```python
from build123d import *

# Parameters (mm, degrees)
BOSS_EXTRUDE1_DEPTH              = 20
F_10_0MM_DOWEL_HOLE1_D           = 10
F_10_0MM_DOWEL_HOLE1_CSINK_D     = 10.05
F_10_0MM_DOWEL_HOLE1_CSINK_ANGLE = 90


with BuildPart() as part:
    # Sketch2 → Boss-Extrude1 (new body)
    with BuildSketch(Plane.XY):
        with BuildLine():
            Line((-15, -240), (-15, 240))
            ThreePointArc((-15, 240), (-7.5, 247.5), (0, 240))
            Line((0, 240), (0, -240))
            ThreePointArc((0, -240), (-7.5, -247.5), (-15, -240))
        make_face()
    extrude(amount=BOSS_EXTRUDE1_DEPTH)

    # Ø10.0mm Dowel Hole1 (through all)
    with Locations(Plane.XY.offset(20)):
        with Locations((-7.5, 240), (-7.5, -240)):
            CounterSinkHole(F_10_0MM_DOWEL_HOLE1_D / 2, F_10_0MM_DOWEL_HOLE1_CSINK_D / 2, counter_sink_angle=F_10_0MM_DOWEL_HOLE1_CSINK_ANGLE)


solid = part.part
```
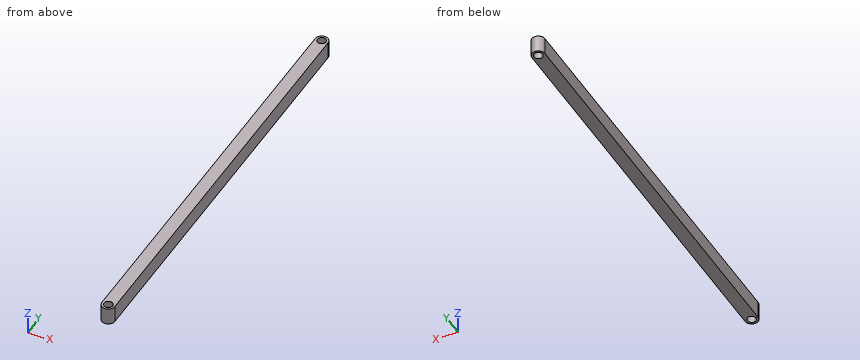
Could you check a few things on this model? Use its own coordinates, in mm. Round coordinates to 2 decimals unless told otherwise and drop trailing zeros. Loops run counter-clockwise (first coordinate to the right, second up) from the corner with the lowest first, then second, coordinate; pieces in that order, holes last.
Q1. I want a section at B-B (z = 3). Write out the boundary of the cut face in (x, y).
Q2. I want a section at A-A (x = -7.5). Write out the boundary of the cut face in (y, z) (3 decimals), and give its area (3 significant figures).
Q3. For P1, Ø4, axis at x = -12.5, z = 10.5, coming from the -Y side; P2, Ø3, axis at x = -2, z = 12.5, coming from the -Y side; P3, Ø8, axis at x = -7.5, y = 240, coming from the -Z side, each with a flat end and sliding along its axis, tell me the tip position at first contact or that it passes through.
Q4. Please list where these lines run through material, in increasing order: L1, parallel to Y at x = -6.75, z = 10.5; L2, parallel to Y at x = -7.5, z = 9.25; L3, parallel to X at y = 240, z = 12.5.
Answer below:
1. outline: (-15, -240) arc R7.5 ccw to (0, -240) - (0, 240) arc R7.5 ccw to (-15, 240) - close; hole circle Ø10 at (-7.5, -240); hole circle Ø10 at (-7.5, 240)
2. outline: (-247.5, 0) - (-245, 0) - (-245, 19.975) - (-245.025, 20) - (-247.5, 20) - close; (-235, 0) - (235, 0) - (235, 19.975) - (234.975, 20) - (-234.975, 20) - (-235, 19.975) - close; (245, 0) - (247.5, 0) - (247.5, 20) - (245.025, 20) - (245, 19.975) - close
2. area: 9,500 mm2
3. P1: stops at y = -246.87
3. P2: stops at y = -246.34
3. P3: passes through
4. L1: y = -247.46 to -244.94, -235.06 to 235.06, 244.94 to 247.46
4. L2: y = -247.5 to -245, -235 to 235, 245 to 247.5
4. L3: x = -15 to -12.5, -2.5 to 0
